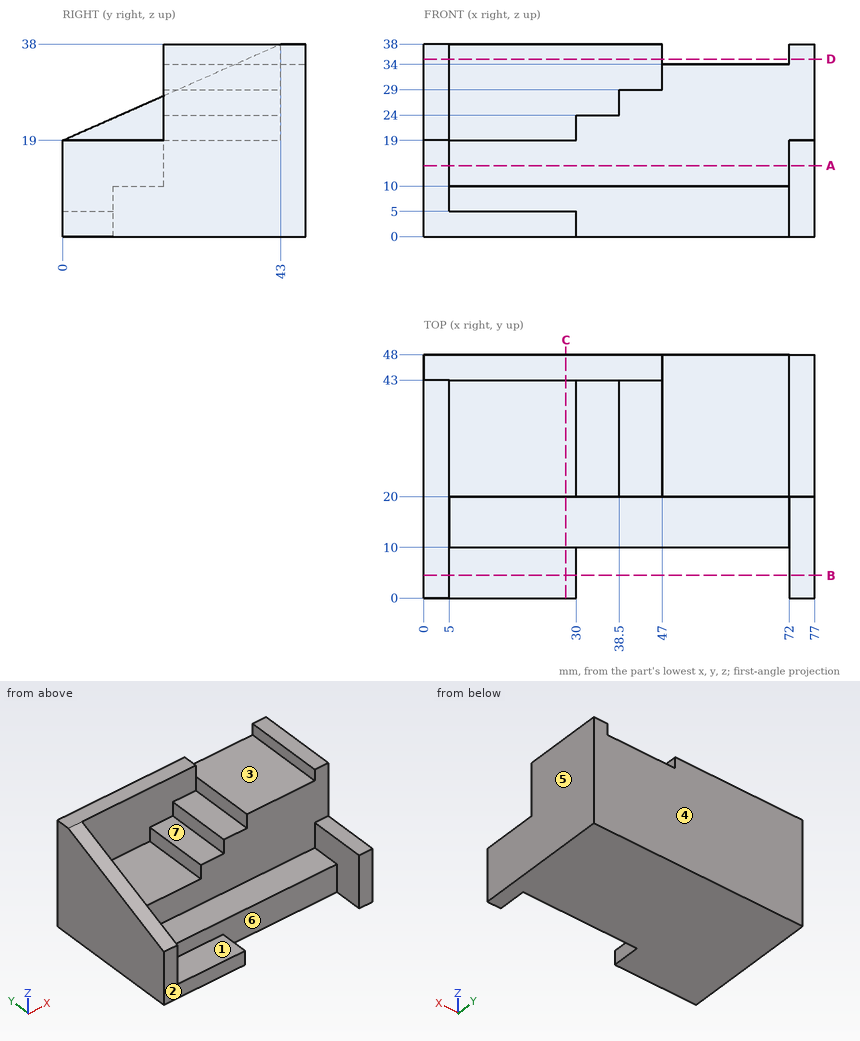
Could you check a few things on this drawing? It's one solid part, dimensions in mm from its lowest x, y, z. A direction names the side the tool comes from. Give positions to 0.01 mm unless a question says otherwise; leave off trailing zeros. Write each loop counter-clockwise with the first axis right and the second up, starting at its lowest first coordinate (ties: lowest second). Pieces come first, ordered by that corner, then holes.
(1) Imagine slicing it at A-A, the plane z = 14. Write out the boundary of the cut face in (x, y), and give its area (3 significant figures).
Output values:
outline: (0, 0) - (5, 0) - (5, 20) - (72, 20) - (72, 0) - (77, 0) - (77, 48) - (0, 48) - close
area: 2,360 mm2
(2) Will these pins go through, and if not, where does the flat tip stop? pin 1 (5 mm diameter, centred on x = 21, y = 6, fed in from +Z); pin 2 (5.5 mm diameter, centred on x = 32, z = 28, fed in from -Y); pin 3 (11 mm diameter, centred on x = 34.5, y = 15.5, fed in from +Z).
Output values:
pin 1: stops at z = 5
pin 2: stops at y = 43
pin 3: stops at z = 24
(3) Imagine slicing it at B-B, the plane y = 4.5. Write out the boundary of the cut face in (x, z).
Output values:
outline: (0, 0) - (30, 0) - (30, 5) - (5, 5) - (5, 20.99) - (0, 20.99) - close; (72, 0) - (77, 0) - (77, 19) - (72, 19) - close
(4) Imagine slicing it at D-D, the plane z = 35. Write out the boundary of the cut face in (x, y).
Output values:
outline: (0, 36.21) - (5, 36.21) - (5, 43) - (47, 43) - (47, 48) - (0, 48) - close; (72, 20) - (77, 20) - (77, 48) - (72, 48) - close
(5) On a 3-axis mill with a long thin cutter (end or side, diameter ignored), from which of +Z, -Z, +X, -X, +Y, -Y can I reach the whole of each face in a straight line? I mean the marked faces 1, 2 and 3. Say none if no direction works.
Output values:
face 1: +Z, -Y
face 2: +Z, -Z, +X, -X, -Y
face 3: +Z, +Y, -Y
(6) Imagine slicing it at C-C, the plane x = 28. Write out the boundary of the cut face in (y, z), and give its area (3 significant figures).
Output values:
outline: (0, 0) - (48, 0) - (48, 38) - (43, 38) - (43, 19) - (20, 19) - (20, 10) - (10, 10) - (10, 5) - (0, 5) - close
area: 777 mm2
(7) If I drill on L1, parallel to X at y = 10.5, z = 18; L2, parallel to X at y = 44.5, z = 35.5; L3, parallel to Z at x = 50.5, y = 44, over which ranges is the centre line in solid material (lowest first)?
Output values:
L1: x = 0 to 5, 72 to 77
L2: x = 0 to 47, 72 to 77
L3: z = 0 to 34
(8) Thinking about a two-plate mould opening in X: for the marked faces 4, 5, 6 and 7, which applies, pulls with the +X half, pulls with the -X half, needs draft (parallel to the pull), parting line crosses it, or undercut?
Output values:
face 4: needs draft
face 5: pulls with the +X half
face 6: undercut
face 7: undercut
